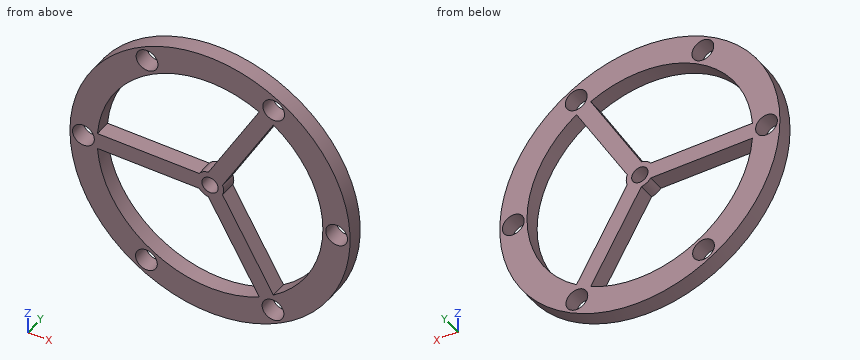
Autodesk Inventor part; units mm, degrees
ref_plane "YZ Plane" through (0, 0, 0) normal (1, 0, 0) x (0, 1, 0)
ref_plane "XZ Plane" through (0, 0, 0) normal (0, 1, 0) x (-1, 0, 0)
ref_plane "XY Plane" through (0, 0, 0) normal (0, 0, 1) x (1, 0, 0)
sketch "Sketch1" plane through (0, 0, 0) normal (0, 1, 0) x (-1, 0, 0)
  circle A0 centre (0, 0) radius 51.45
  circle A1 centre (0, 0) radius 3
  line L0 (4, -3) -> (43.45, -3)
  line L1 (0.5981, 4.9641) -> (-19.1269, 39.1288)
  line L2 (-4.5981, -1.9641) -> (-24.3231, -36.1288)
  line L3 (4, 3) -> (43.45, 3)
  line L4 (-4.5981, 1.9641) -> (-24.3231, 36.1288)
  line L5 (0.5981, -4.9641) -> (-19.1269, -39.1288)
  arc A2 (4, 3) -> (0.5981, 4.9641) centre (0, 0) ccw
  arc A3 (-4.5981, 1.9641) -> (-4.5981, -1.9641) centre (0, 0) ccw
  arc A4 (0.5981, -4.9641) -> (4, -3) centre (0, 0) ccw
  arc A5 (-23.2687, 34.3026) -> (-23.2687, -34.3026) centre (0, 0) ccw
  arc A6 (-18.0726, -37.3026) -> (41.3413, -3) centre (0, 0) ccw
  arc A7 (41.3413, 3) -> (-18.0726, 37.3026) centre (0, 0) ccw
  circle A8 centre (-23.127, -40.341) radius 4
  circle A9 centre (23.3728, -40.199) radius 4
  circle A10 centre (46.4998, 0.1419) radius 4
  circle A11 centre (23.127, 40.341) radius 4
  circle A12 centre (-23.3728, 40.199) radius 4
  circle A13 centre (-46.4998, -0.1419) radius 4
  dimension "d0" = 102.9
  dimension "d2" = 6
  dimension "d7" = 360
  dimension "d9" = 6
  dimension "d12" = 360
  dimension "d16" = 8
  dimension "d17" = 46.5
  dimension "d20" = 360
extrude "Extrusion2" add sketch "Sketch1" along normal blind 6
properties part number "reaction wheel" material "PC/ABS Plastic"
Build history of the part. All positions in model axes, mm. Give positions to 0.01 mm unless a question says otherwise; leave off trailing zeros. Order: outer loops, then holes, each group sorted by start corner. A loop starts at its lowest first (then second) coordinate and runs counter-clockwise, first axis right, second up. Notation, with made-up numbers: M 47.25,55 L 79.25,55 A26 ccw 79.25,75 Z; hole C 18,-3 d6. An arc over 180 degrees is marked long. Use one line per item in the form item = value.
1) Saw through at D-D (y = 3.8). State how many separate pieces and enclosed holes the cut face has, plus the area to 3 significant figures.
Calculated:
separate_pieces = 1
enclosed_holes = 10
area = 3,330 mm2
2) Saw through at B-B (x = -29). Give the cut face in (y, z).
Calculated:
outline = M 0,-42.5 L 6,-42.5 L 6,-29.62 L 0,-29.62 Z; M 0,-3 L 6,-3 L 6,3 L 0,3 Z; M 0,29.62 L 6,29.62 L 6,42.5 L 0,42.5 Z
3) Probe probe 1 along Z at (x, y) = (18, 3.05); probe 2 along X at (y, z) = (2.35, 28); probe 3 along X at (y, z) = (4.95, 34). List the from-to ranges inside material, lowest first.
Calculated:
probe_1 = -48.2 to -37.34, -37.18 to -25.18, 25.18 to 37.18, 37.34 to 48.2
probe_2 = -43.16 to -30.56, 12.7 to 19.63, 30.56 to 43.16
probe_3 = -38.61 to -23.71, 16.17 to 23.09, 23.71 to 38.61
4) Saw through at C-C (x = 6.5). Give the cut face in (y, z), plus the area to 3 significant figures.
Calculated:
outline = M 0,-51.04 L 6,-51.04 L 6,-40.94 L 0,-40.94 Z; M 0,-17.26 L 6,-17.26 L 6,-5.26 L 0,-5.26 Z; M 0,5.26 L 6,5.26 L 6,17.26 L 0,17.26 Z; M 0,40.94 L 6,40.94 L 6,51.04 L 0,51.04 Z
area = 265 mm2
5) Saw through at A-A (z = 29). Give the cut face in (x, y), plus the area to 3 significant figures.
Calculated:
outline = M -42.5,0 L -29.62,0 L -29.62,6 L -42.5,6 Z; M 13.28,0 L 20.21,0 L 20.21,6 L 13.28,6 Z; M 29.62,0 L 42.5,0 L 42.5,6 L 29.62,6 Z
area = 196 mm2
6) Drop flat-ended pins along their axis: pin 1 (1 mm diameter, centred on x = -12, y = 3, fed in from +Z); pin 2 (2 mm diameter, centred on y = 1, z = 7.5, fed in from +X); pin 3 (7 mm diameter, centred on x = 23.127, z = -40.341, fed in from -Y); pin 4 (3 mm diameter, centred on x = -24, y = 2.5, fed in from +Z). Give the stop position or say it passes through.
Calculated:
pin_1 = 50.15
pin_2 = 51.04
pin_3 = through
pin_4 = 46.27
